from build123d import *

# Parameters (mm, degrees)
SKETCH1_W           = 48
SKETCH1_H           = 48
BOSS_EXTRUDE1_DEPTH = 80
SKETCH2_W           = 48
SKETCH2_H           = 48
BOSS_EXTRUDE2_DEPTH = 15
FILLET2_R           = 24
SKETCH3_R           = 5
BOSS_EXTRUDE3_DEPTH = 7.5
SKETCH4_R           = 5
BOSS_EXTRUDE4_DEPTH = 7.5


with BuildPart() as part:
    # Sketch1 → Boss-Extrude1 (new body)
    with BuildSketch(Plane(origin=(0, 0, 0), x_dir=(1, 0, 0), z_dir=(0, 1, 0))):
        with Locations((24, 24)):
            Rectangle(SKETCH1_W, SKETCH1_H)
    extrude(amount=BOSS_EXTRUDE1_DEPTH)

    # Sketch2 → Boss-Extrude2 (add)
    with BuildSketch(Plane(origin=(48, 0, 0), x_dir=(0, 0, -1), z_dir=(1, 0, 0))):
        with Locations((24, 56)):
            Rectangle(SKETCH2_W, SKETCH2_H)
    extrude(amount=BOSS_EXTRUDE2_DEPTH)

    # Fillet2
    fillet2_edges = [part.edges().sort_by_distance(p)[0] for p in [
        (48, 16, -48),
        (48, 16, 0),
        (55.5, 32, 0),
        (31.5, 80, -48),
        (55.5, 32, -48),
        (0, 80, -24),
        (0, 40, -48),
        (0, 40, 0),
        (31.5, 80, 0),
    ]]
    fillet(fillet2_edges, radius=FILLET2_R - 0.0001)  # a hair under: the kernel refuses the full size

    # Sketch3 → Boss-Extrude3 (add, symmetric)
    with BuildSketch(Plane(origin=(0, 0, 0), x_dir=(-1, 0, 0), z_dir=(0, -1, 0))):
        with Locations(Location((-24, 24, 0), (0, 0, 90))):
            Circle(SKETCH3_R)
    extrude(amount=BOSS_EXTRUDE3_DEPTH, both=True)

    # Sketch4 → Boss-Extrude4 (add, symmetric)
    with BuildSketch(Plane(origin=(63, 0, 0), x_dir=(0, 0, -1), z_dir=(1, 0, 0))):
        with Locations((24, 56)):
            Circle(SKETCH4_R)
    extrude(amount=BOSS_EXTRUDE4_DEPTH, both=True)


solid = part.part
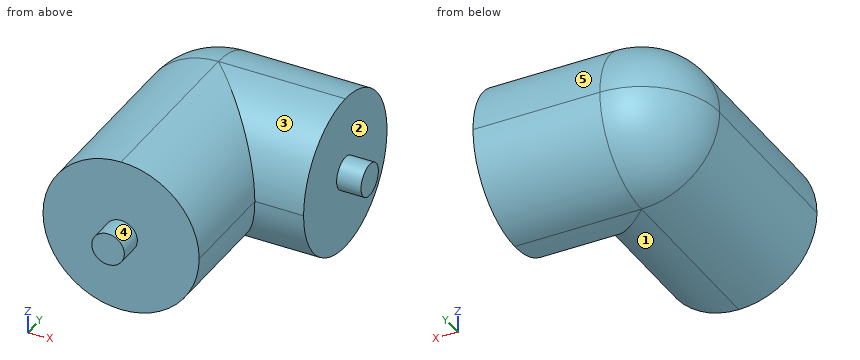
Can you work these out from the model? Positions are in its coordinate system, mm. Face numbers are marked on the shaded views. A direction names the side the tool comes from. Give positions to 0.01 mm unless a question says otherwise; leave off trailing zeros. Order: outer loops, then holes, each group sorted by start corner. A loop starts at its lowest first (then second) coordinate and runs counter-clockwise, first axis right, second up. Notation, with made-up numbers: M 34.25,41.5 L 48.25,41.5 A15 cw 48.25,48.5 Z; hole C -24,33.25 d1. An arc over 180 degrees is marked long. One line per question, with ' | ' between items.
Item 1: I'm going to push flat-ended pins straight in: pin 1 Ø1.5 at (x, y) = (38, 51.5) entering from +Z; pin 2 Ø2 at (y, z) = (26.5, -38) entering from -X; pin 3 Ø1.5 at (x, z) = (63.5, -27.5) entering from -Y. Where does each tip first touch, or does it pass through?
Answer block:
pin 1: stops at z = -0.29 | pin 2: stops at x = 3.83 | pin 3: stops at y = 32.18
Item 2: For the marked faces 1, 2, 3, 4 and 5, which set-ups out of +Z, -Z, +X, -X, +Y, -Y let a thin tool reach every point of the face, with its end or its side?
Answer block:
face 1: -Z, +X, -Y | face 2: +X | face 3: +Z, +X, -Y | face 4: -Y | face 5: +Z, +X, -X, +Y
Item 3: Suppose I cut it at A-A, the plane z = -21. Write out the boundary of the cut face in (x, y), then the cut area to 3 significant figures.
Answer block:
outline: M 0.19,0 L 20,0 L 20,-7.5 L 28,-7.5 L 28,0 L 47.81,0 L 47.81,32.19 L 63,32.19 L 63,52 L 70.5,52 L 70.5,60 L 63,60 L 63,79.81 L 24,79.81 A23.81 ccw 0.19,56 Z | area: 4,520 mm2
Item 4: Suppose I cut it at D-D, the plane z = -3. Write out the boundary of the cut face in (x, y).
Answer block:
outline: M 12.38,0 L 35.62,0 L 35.62,44.38 L 63,44.38 L 63,67.62 L 24,67.62 A11.62 ccw 12.38,56 Z
Item 5: Please list where these lines run through material, in increasing order: L1, parallel to Z at x = 50, y = 57; L2, parallel to X at y = 46.5, z = -17; L3, parallel to X at y = 46, z = -2.
Answer block:
L1: z = -47.98 to -0.02 | L2: x = 1.04 to 63 | L3: x = 14.41 to 33.59
